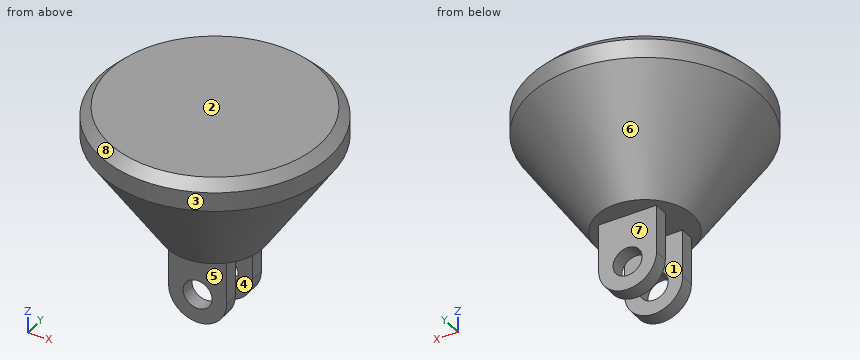
from build123d import *

# Parameters (mm, degrees)
F2_DEPTH = 6
F3_DEPTH = 3
F4_SIZE  = 2
F6_D     = 6


with BuildPart() as f1:
    # F0 (on Front) → F1 (revolve)
    with BuildSketch(Plane.XZ):
        Polygon((-6, 0), (0, 0), (0, 27), (-24, 27), (-24, 21), (-10, 0), align=None)
    revolve(axis=Axis((0, 0, 13.5), (0, 0, 1)))

    # F0 (on Front) → F2 (join, symmetric)
    with BuildSketch(Plane.XZ):
        with BuildLine():
            Line((6, 0), (0, 0))
            Line((0, 0), (-6, 0))
            Line((-6, 0), (-6, -10))
            ThreePointArc((-6, -10), (0, -16), (6, -10))
            Line((6, -10), (6, 0))
        make_face()
    extrude(amount=F2_DEPTH, both=True)

    # F0 (on Front) → F3 (cut, symmetric)
    with BuildSketch(Plane.XZ):
        with BuildLine():
            Line((6, 0), (0, 0))
            Line((0, 0), (-6, 0))
            Line((-6, 0), (-6, -10))
            ThreePointArc((-6, -10), (0, -16), (6, -10))
            Line((6, -10), (6, 0))
        make_face()
    extrude(amount=F3_DEPTH, both=True, mode=Mode.SUBTRACT)

    # F4
    f4_edges = [f1.edges().sort_by_distance(p)[0] for p in [
        (24, 0, 27),
    ]]
    chamfer(f4_edges, length=F4_SIZE)

    # F6 (through all)
    with Locations(Plane.XZ.offset(6)):
        with Locations((0, -10)):
            Hole(F6_D / 2)


solid = f1.part
Design review of the part built by this model. Coordinates are the model's own, in mm. Face numbers are marked on the shaded views. A direction names the side the tool comes from. Round coordinates to 2 decimals unless told otherwise and drop trailing zeros. Write each loop counter-clockwise with the first axis right and the second up, starting at its lowest first coordinate (ties: lowest second). Pieces come first, ordered by that corner, then holes. Notation, with made-up numbers: (-30.5, 75) - (-0.5, 75) arc R23 cw to (-0.5, 108) - close; hole circle Ø2 at (5.25, 2). An arc over 180 degrees is marked (long way). Use a Markdown table: item, result. Add a question column.
1. We need section D-D (z = 18). State the section outline as (x, y) points.
2. We need section B-B (z = -3). State the section outline as (x, y) points, then the cut area to 3 significant figures.
3. Clearance check with flat-ended pins moving along their axes: pin 1 (8 mm diameter, centred on x = 0, z = -10, fed in from +Y); pin 2 (8 mm diameter, centred on x = 5, z = 3, fed in from +Y); pin 3 (6 mm diameter, centred on x = -12, y = -15, fed in from -Z); pin 4 (3.5 mm diameter, centred on x = 0, z = -10, fed in from -Y). State where each tip first meets the part, or that it passes through.
4. We need section C-C (y = 0). State the section outline as (x, z) points.
5. We need section A-A (x = 0). State the section outline as (y, z) points, then the cut area to 3 significant figures.
6. Mouldability with a two-part tool opening along Y and no side actions: class the marked faces 1, 2 and 3 as +Y half, -Y half, draft (parallel to the pull), parting line (faces both ways), or undercut.
7. Wall thickness on probe 1 along Z at (x, y) = (0, 4); probe 2 along Y at (x, z) = (3.5, -11); probe 3 along Z at (x, y) = (0, 7): over which ranges is each line inside the solid? List them lowest first.
8. For the marked faces 4, 5, 6, 7 and 8, list the 3-axis set-ups (+Z, -Z, +X, -X, +Y, -Y) from which the entire face can be reached by the end or side of a thin tool; tool diameter is ignored.
Output:
| question | item | result |
|---|---|---|
| 1 | outline | circle Ø44 at (0, 0) |
| 2 | outline | (-6, -6) - (6, -6) - (6, -3) - (-6, -3) - close; (-6, 3) - (6, 3) - (6, 6) - (-6, 6) - close |
| 2 | area | 72.0 mm2 |
| 3 | pin 1 | stops at y = 6 |
| 3 | pin 2 | stops at y = 14.04 |
| 3 | pin 3 | stops at z = 9.31 |
| 3 | pin 4 | passes through |
| 4 | outline | (-24, 21) - (-10, 0) - (10, 0) - (24, 21) - (24, 25) - (22, 27) - (-22, 27) - (-24, 25) - close |
| 5 | outline | (-24, 21) - (-10, 0) - (-6, 0) - (-6, -7) - (-3, -7) - (-3, 0) - (3, 0) - (3, -7) - (6, -7) - (6, 0) - (10, 0) - (24, 21) - (24, 25) - (22, 27) - (-22, 27) - (-24, 25) - close; (-6, -16) - (-3, -16) - (-3, -13) - (-6, -13) - close; (3, -16) - (6, -16) - (6, -13) - (3, -13) - close |
| 5 | area | 1,060 mm2 |
| 6 | face 1 | undercut |
| 6 | face 2 | draft |
| 6 | face 3 | parting line |
| 7 | probe 1 | z = -16 to -13, -7 to 27 |
| 7 | probe 2 | y = -6 to -3, 3 to 6 |
| 7 | probe 3 | z = 0 to 27 |
| 8 | face 4 | -Z, +X, -X |
| 8 | face 5 | -Z, +X, -X, -Y |
| 8 | face 6 | -Z |
| 8 | face 7 | -Z, +X, -X, +Y |
| 8 | face 8 | +Z |
